For this review, take the finished solid that the model builds, in its own axes (mm). A direction names the side the tool comes from. Give positions to 0.01 mm unless a question says otherwise; leave off trailing zeros. Write each loop counter-clockwise with the first axis right and the second up, starting at its lowest first coordinate (ties: lowest second). Pieces come first, ordered by that corner, then holes. Notation, with made-up numbers: (-1, 23) -> (33, 23) arc R15 cw to (33, 45) -> close; hole circle Ø5 at (-12, 36.5). An arc over 180 degrees is marked (long way). Answer as CSV lines item,"result".
```python
from build123d import *

# Parameters (mm, degrees)
SHELL1_T           = -2.54
CUT_EXTRUDE1_REACH = 151.86
SKETCH2_R          = 12.7


with BuildPart() as part:
    # Sketch1 → Revolve1 (revolve)
    with BuildSketch(Plane.XY):
        Polygon((0, 0), (0, 353.06), (149.86, 353.06), (130.048, 0), align=None)
    revolve(axis=Axis((0, 0, 0), (0, 1, 0)))

    # Shell1
    shell1_openings = [part.faces().sort_by_distance(p)[0] for p in [
        (0, 353.06, -149.86),
    ]]
    offset(amount=SHELL1_T, openings=shell1_openings, kind=Kind.INTERSECTION)

    # Sketch2 → Cut-Extrude1 (cut, up to next)
    with BuildSketch(Plane.XY, mode=Mode.PRIVATE) as cut_extrude1_sk1:
        with Locations((0, 42.17291268)):
            Circle(SKETCH2_R)
    cut_extrude1_tool1 = extrude(cut_extrude1_sk1.sketch, amount=CUT_EXTRUDE1_REACH, mode=Mode.PRIVATE) & part.part
    add(cut_extrude1_tool1.solids().sort_by_distance((0, 42.172913, 0))[0], mode=Mode.SUBTRACT)


solid = part.part
```
Q1. Draft analysis for pull direction Y (two halves, no side actions). For faces 3 (the cylindrical face through (5.86, 30.906, 130.602)), 4 (the conical face through (131.001, 175.346, -41.254)), 5 (the conical face through (-30.31, 174.06, 136.49)), state which applies: released by +Y, released by -Y, zero draft, split by the parting line, or undercut.
Answer block:
face 3,"undercut"
face 4,"released by +Y"
face 5,"released by -Y"
Q2. For faces 1 (the flat face through (-2, 2.54, -2)), 2 (the flat face through (-110, 353.06, 99)), list the 3-axis set-ups (+Z, -Z, +X, -X, +Y, -Y) from which the entire face can be reached by the end or side of a thin tool; tool diameter is ignored.
Answer block:
face 1,"+Y"
face 2,"+Z, -Z, +X, -X, +Y"
Q3. Add section C-C (y = 220.5). Write out the cut boundary in (x, z), plus the area to 3 significant figures.
Answer block:
outline,"circle Ø284.84 at (0, 0); hole circle Ø279.75 at (0, 0)"
area,"2,260 mm2"
Q4. Add section D-D (y = 157.5). Write out the cut boundary in (x, z), plus the area to 3 significant figures.
Answer block:
outline,"circle Ø277.77 at (0, 0); hole circle Ø272.68 at (0, 0)"
area,"2,200 mm2"
Q5. Clearance check with flat-ended pins moving along their axes: pin 1 (3 mm diameter, centred on x = 96.5, y = 292, fed in from -Z); pin 2 (4 mm diameter, centred on x = 92.5, y = 181, fed in from -Z); pin 3 (10 mm diameter, centred on x = 71.5, y = 68, fed in from -Z). State where each tip first meets the part, or that it passes through.
Answer block:
pin 1,"stops at z = -111.44"
pin 2,"stops at z = -107.09"
pin 3,"stops at z = -116.2"
Q6. Add section B-B (z = 0). Write out the cut boundary in (x, y), plus the area to 3 significant figures.
Answer block:
outline,"(-149.86, 353.06) -> (-130.05, 0) -> (130.05, 0) -> (149.86, 353.06) -> (147.32, 353.06) -> (127.65, 2.54) -> (-127.65, 2.54) -> (-147.32, 353.06) -> close"
area,"2,440 mm2"
Q7. To check wall thickness, follow probe 1 along Z at (x, y) = (48.5, 284); probe 2 along X at (y, z) = (208, 127); probe 3 along X at (y, z) = (333.5, -95). State the ranges of each line that lie inside material, in increasing order. Write a range as [from, to].
Answer block:
probe 1,"z = [-137.69, -134.99], [134.99, 137.69]"
probe 2,"x = [-62.89, -56.93], [56.93, 62.89]"
probe 3,"x = [-114.48, -111.15], [111.15, 114.48]"
Q8. Add section A-A (x = 0). Write out the cut boundary in (y, z).
Answer block:
outline,"(0, -130.05) -> (353.06, -149.86) -> (353.06, -147.32) -> (2.54, -127.65) -> (2.54, 127.65) -> (29.47, 129.16) -> (29.47, 131.7) -> (0, 130.05) -> close; (54.87, 130.58) -> (353.06, 147.32) -> (353.06, 149.86) -> (54.87, 133.13) -> close"
